For this review, take the finished solid that the model builds, in its own axes (mm). A direction names the side the tool comes from. Round coordinates to 2 decimals unless told otherwise and drop trailing zeros. Order: outer loops, then holes, each group sorted by start corner. A loop starts at its lowest first (then second) coordinate and runs counter-clockwise, first axis right, second up. Notation, with made-up numbers: (5.25, 48) - (48.25, 48) arc R24 cw to (48.25, 59) - close; hole circle Ø7 at (3, 62.25). An arc over 180 degrees is marked (long way). One line per item, written item: value.
```python
from build123d import *

# Parameters (mm, degrees)
SKETCH_2_W          = 95
SKETCH_2_H          = 12
EXTRUDE_2_DEPTH     = 12
SKETCH_7_W          = 12
SKETCH_7_H          = 95
EXTRUDE_6_DEPTH     = 12
SKETCH_5_RX         = 20
SKETCH_5_RY         = 7
SKETCH_5_RY_2       = 7.000177109
EXTRUDE_5_DEPTH     = 12
CUT_EXTRUDE_1_DEPTH = 10.5
FILLET_1_R          = 10
SKETCH_9_R          = 1.5
CUT_EXTRUDE_2_DEPTH = 82.992066392


with BuildPart() as part:
    # 草图2 → 凸台-拉伸2 (new body)
    with BuildSketch(Plane.XY):
        Rectangle(SKETCH_2_W, SKETCH_2_H)
    extrude(amount=EXTRUDE_2_DEPTH)

    # 草图7 → 凸台-拉伸6 (add)
    with BuildSketch(Plane.XY.offset(12)):
        Rectangle(SKETCH_7_W, SKETCH_7_H)
    extrude(amount=-EXTRUDE_6_DEPTH)

    # 草图5 → 凸台-拉伸5 (add)
    with BuildSketch(Plane(origin=(0, 0, 0), x_dir=(-1, 0, 0), z_dir=(0, 0, -1))):
        with Locations(Location((-37.5, 0), (0, 0, 0))):
            Ellipse(SKETCH_5_RX, SKETCH_5_RY)
        with Locations(Location((0, 37.5), (0, 0, 90.407571877))):
            Ellipse(SKETCH_5_RX, SKETCH_5_RY_2)
        with Locations(Location((37.5, 0), (0, 0, 0.407571877))):
            Ellipse(SKETCH_5_RX, SKETCH_5_RY_2)
        with Locations(Location((0, -37.5), (0, 0, -89.592428123))):
            Ellipse(SKETCH_5_RX, SKETCH_5_RY_2)
    extrude(amount=-EXTRUDE_5_DEPTH)

    # 草图8 → 切除-拉伸1 (cut)
    with BuildSketch(Plane.XY.offset(12)):
        with BuildLine():
            ThreePointArc((2.8, 0), (0.836660027, 2.672077843), (-2.3, 1.596871942))
            Line((-2.3, 1.596871942), (-2.3, -1.596871942))
            ThreePointArc((-2.3, -1.596871942), (0.836660027, -2.672077843), (2.8, 0))
        make_face()
    extrude(amount=-CUT_EXTRUDE_1_DEPTH, mode=Mode.SUBTRACT)

    # 圆角1
    fillet_1_edges = [part.edges().sort_by_distance(p)[0] for p in [
        (6, 6, 6),
        (6, -6, 6),
        (-6, 6, 6),
        (-6, -6, 6),
    ]]
    fillet(fillet_1_edges, radius=FILLET_1_R)

    # 草图9 → 切除-拉伸2 (cut, through all)
    with BuildSketch(Plane.XY.offset(1.5)):
        Circle(SKETCH_9_R)
    extrude(amount=-CUT_EXTRUDE_2_DEPTH, mode=Mode.SUBTRACT)


solid = part.part
```
Item 1: For P1, Ø5.5, axis at x = -19.5, z = 3.5, coming from the -Y side; P2, Ø5.5, axis at x = 23, z = 3, coming from the +Y side; P3, Ø1.5, axis at y = -40.5, z = 8, coming from the -X side, all flat-tipped, find the tip position at first contact; note any pin that passes through.
Returned:
P1: y = -6
P2: y = 6
P3: x = -6.97
Item 2: Take a section at B-B (y = 12). Write out the cut boundary in (x, z), plus the area to 3 significant figures.
Returned:
outline: (-6.83, 0) - (6.83, 0) - (6.83, 12) - (-6.83, 12) - close
area: 164 mm^2
Item 3: Machinability: for faces 5 (the flat face through (6, -22, 6)), 6 (the flat face through (22, 6, 6)), 7 (the flat face through (-6, 21, 6)), 8 (the flat face through (-2.3, 0, 7)), which of the approach directions +Z, -Z, +X, -X, +Y, -Y give a long, thin tool a straight path to every point of the face, cutting with its end or side? Answer none if there is none.
Returned:
face 5: +Z, -Z, +X
face 6: +Z, -Z, +Y
face 7: +Z, -Z, -X
face 8: +Z
Item 4: The part is to be moulded in two halves that separate along Y. For faces 1 (the flat face through (-22, -6, 6)), 2 (the cylindrical face through (9.01, 8.85, 5.92)), 3 (the flat face through (6, 22, 6)), 4 (the flat face through (4, 0, 12)), say which applies: +Y half, -Y half, draft (parallel to the pull), parting line (faces both ways), or undercut.
Returned:
face 1: -Y half
face 2: undercut
face 3: undercut
face 4: draft
Item 5: Wall thickness on line 1 (Y direction, x = 0, z = 1); line 2 (X direction, y = 26, z = 3.5); line 3 (Y direction, x = 37, z = 4.25): over which ranges is each line inside the solid? List them lowest first.
Returned:
line 1: -57.5 to -1.5, 1.5 to 57.5
line 2: -6 to 6
line 3: -7 to 7
Item 6: Take a section at A-A (x = 17.5). Write out the cut boundary in (y, z).
Returned:
outline: (-6, 0) - (6, 0) - (6, 12) - (-6, 12) - close
